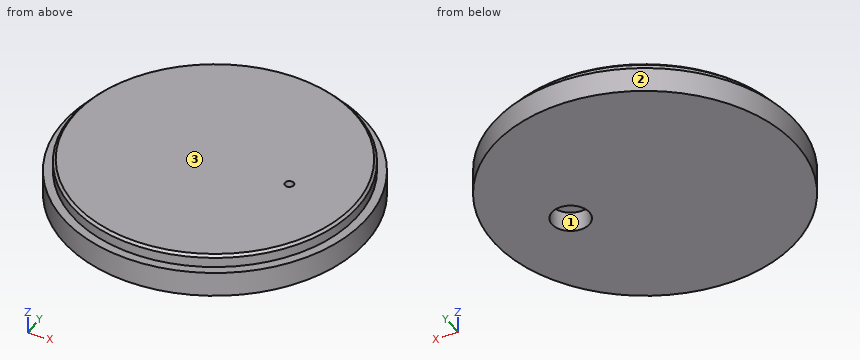
from build123d import *

# Parameters (mm, degrees)
SKETCH_R        = 57
PAD_DEPTH       = 5
SKETCH001_R     = 60.5
PAD001_DEPTH    = 10
CHAMFER_SIZE    = 1
SKETCH002_R     = 1.75
POCKET_DEPTH    = 15.001
SKETCH003_R     = 7.5
POCKET001_DEPTH = 8


with BuildPart() as part:
    # Sketch → Pad (new body)
    with BuildSketch(Plane.XY):
        Circle(SKETCH_R)
    extrude(amount=PAD_DEPTH)

    # Sketch001 (on Face2 of Pad) → Pad001 (join)
    with BuildSketch(Plane(origin=(0, 0, 0), x_dir=(1, 0, 0), z_dir=(0, 0, -1))):
        Circle(SKETCH001_R)
    extrude(amount=PAD001_DEPTH)

    # Chamfer
    chamfer_edges = [part.edges().sort_by_distance(p)[0] for p in [
        (-57, 0, 5),
    ]]
    chamfer(chamfer_edges, length=CHAMFER_SIZE)

    # Sketch002 (on Face4 of Chamfer) → Pocket (cut, through all)
    with BuildSketch(Plane.XY.offset(5)):
        with Locations((30, 0)):
            Circle(SKETCH002_R)
    extrude(amount=-POCKET_DEPTH, mode=Mode.SUBTRACT)

    # Sketch003 (on Face7 of Pocket) → Pocket001 (cut)
    with BuildSketch(Plane(origin=(0, 0, -10), x_dir=(1, 0, 0), z_dir=(0, 0, -1))):
        with Locations((30, 0)):
            Circle(SKETCH003_R)
    extrude(amount=-POCKET001_DEPTH, mode=Mode.SUBTRACT)


solid = part.part
Read the model definition and answer for the solid it produces. Units are mm, in the model's axes. Face numbers are marked on the shaded views. Coordinates: 2 decimals unless noted, no trailing zeros. Order: outer loops, then holes, each group sorted by start corner. A loop starts at its lowest first (then second) coordinate and runs counter-clockwise, first axis right, second up. Notation, with made-up numbers: (59, 64.5) - (94, 64.5) arc R16 cw to (94, 87.5) - close; hole circle Ø6 at (-19, -16). An arc over 180 degrees is marked (long way). Use one line per item in the form item = value.
(1) Given pin 1 Ø2 at (y, z) = (45.5, -1) entering from +X; pin 2 Ø1 at (x, z) = (6.5, -3) entering from -Y; pin 3 Ø1.5 at (y, z) = (-9.5, -4) entering from +X, each flat-ended and moving along its own axis, determine where each tip first touches the part or whether it passes through.
Computed values:
pin_1 = 40.99
pin_2 = -60.2
pin_3 = 59.86
(2) Section A-A, the plane y = 0 is taken. Give the vertices of the cut face in (x, z), then the cut area to 3 significant figures.
Computed values:
outline = (-60.5, -10) - (22.5, -10) - (22.5, -2) - (28.25, -2) - (28.25, 5) - (-56, 5) - (-57, 4) - (-57, 0) - (-60.5, 0) - close; (31.75, -2) - (37.5, -2) - (37.5, -10) - (60.5, -10) - (60.5, 0) - (57, 0) - (57, 4) - (56, 5) - (31.75, 5) - close
area = 1,630 mm²
(3) Straight lines are drawn through the part: L1, parallel to X at y = 0, z = -6; L2, parallel to Z at x = 29, y = 2; L3, parallel to Y at x = 30, z = 2.25. For each, find the intervals that lie inside material, in ascending order.
Computed values:
L1 = -60.5 to 22.5, 37.5 to 60.5
L2 = -2 to 5
L3 = -48.47 to -1.75, 1.75 to 48.47
(4) Section C-C, the plane x = 0 is taken. Give the vertices of the cut face in (y, z).
Computed values:
outline = (-60.5, -10) - (60.5, -10) - (60.5, 0) - (57, 0) - (57, 4) - (56, 5) - (-56, 5) - (-57, 4) - (-57, 0) - (-60.5, 0) - close
(5) Section B-B, the plane z = 2.5 is taken. Give the vertices of the cut face in (x, y).
Computed values:
outline = circle Ø114 at (0, 0); hole circle Ø3.5 at (30, 0)
(6) For a pull along Y with two mould halves and no side action, classify the marked faces 1, 2 and 3 as pulls with the +Y half, pulls with the -Y half, needs draft (parallel to the pull), parting line crosses it, or undercut.
Computed values:
face_1 = undercut
face_2 = parting line crosses it
face_3 = needs draft
(7) Section D-D, the plane z = -4 is taken. Give the vertices of the cut face in (x, y).
Computed values:
outline = circle Ø121 at (0, 0); hole circle Ø15 at (30, 0)
